Design review of the part shown in the three views and the two pictorial views. Dimensions are in mm from the part's minimum x, y and z. Round coordinates to 2 decimals unless told otherwise and drop trailing zeros. Loops run counter-clockwise (first coordinate to the right, second up) from the corner with the lowest first, then second, coordinate; pieces in that order, holes last. Notation, with made-up numbers: (67.5, 76.5) -> (122.5, 76.5) arc R21 cw to (122.5, 102.5) -> close; hole circle Ø4 at (-29.75, 32). An arc over 180 degrees is marked (long way). Use a Markdown table: item, result. Add a question column.
1) Insertion check: pin 1 (1.5 mm diameter, centred on x = 45.5, z = 32.5, fed in from +Y); pin 2 (6 mm diameter, centred on y = 14, z = 9.5, fed in from +X); pin 3 (2 mm diameter, centred on x = 34.5, z = 33, fed in from -Y). Each pin has a flat end and moves straight along its axis. Give the tip position at first contact, or say it passes through.
2) Consider section A-A on x = 44.45. Give the boundary of the cut face in (y, z), plus the area to 3 significant figures.
3) Wall thickness on probe 1 along X at (y, z) = (44.5, 50); probe 2 along X at (y, z) = (23, 55.5): over which ranges is each line inside the solid? List them lowest first.
4) Consider section C-C on z = 67. Give the boundary of the cut face in (x, y), plus the area to 3 significant figures.
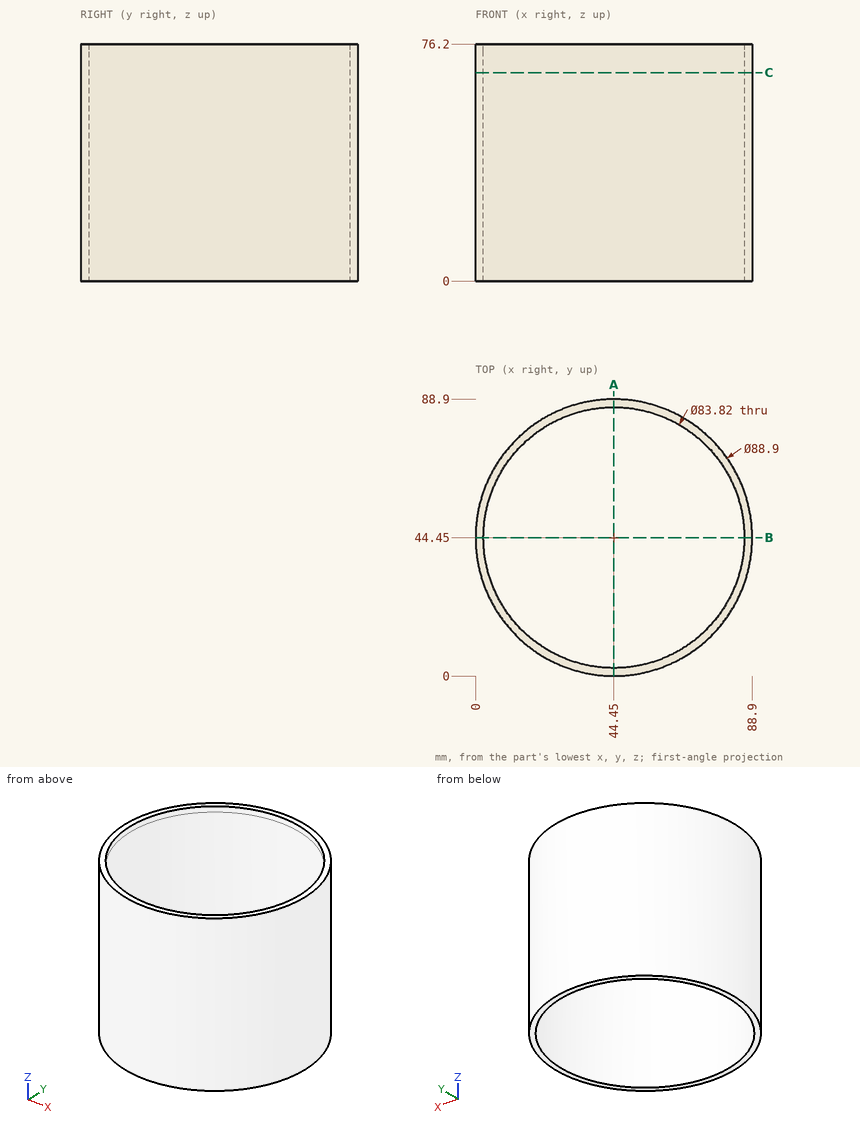
Result set:
| question | item | result |
|---|---|---|
| 1 | pin 1 | y = 88.9 |
| 1 | pin 2 | x = 79.41 |
| 1 | pin 3 | y = 0.91 |
| 2 | outline | (0, 0) -> (2.54, 0) -> (2.54, 76.2) -> (0, 76.2) -> close; (86.36, 0) -> (88.9, 0) -> (88.9, 76.2) -> (86.36, 76.2) -> close |
| 2 | area | 387 mm2 |
| 3 | probe 1 | 0 to 2.54, 86.36 to 88.9 |
| 3 | probe 2 | 5.52 to 8.45, 80.45 to 83.38 |
| 4 | outline | circle Ø88.9 at (44.45, 44.45); hole circle Ø83.82 at (44.45, 44.45) |
| 4 | area | 689 mm2 |
